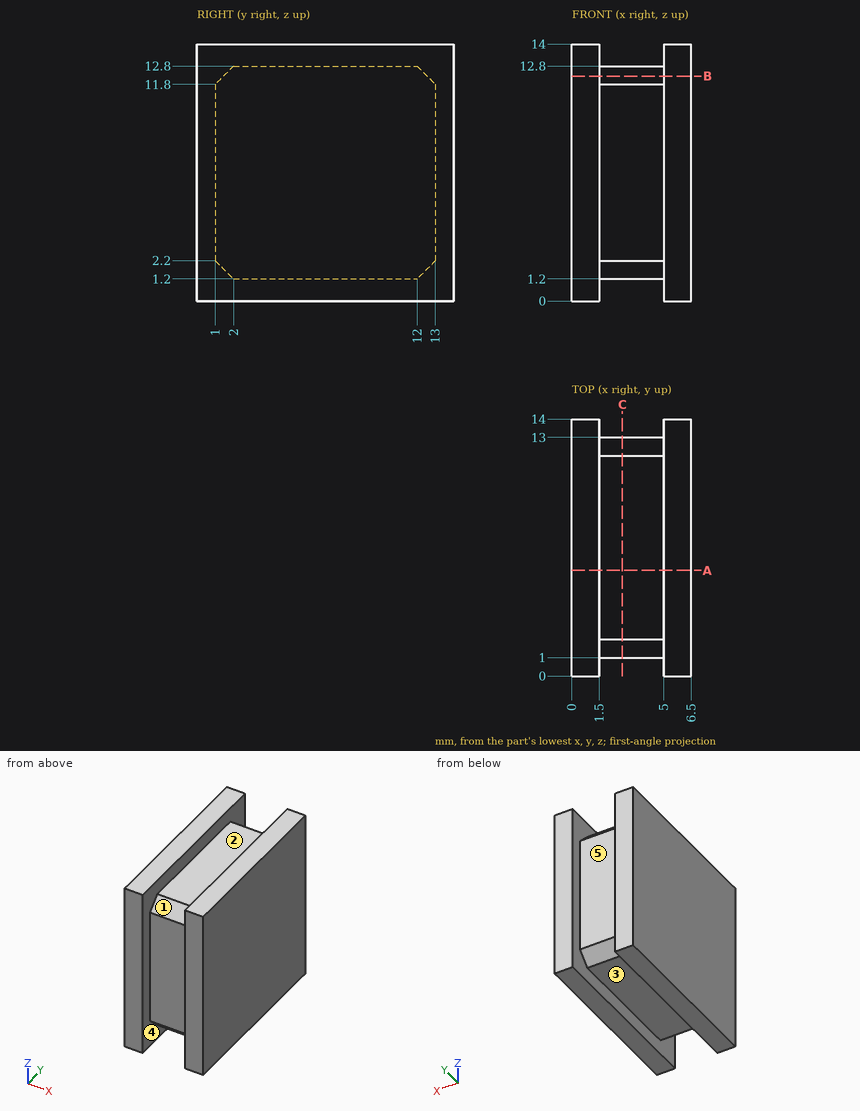
Drawing for the job (mm, zero at the part's lowest x, y, z). A direction names the side the tool comes from. Round coordinates to 2 decimals unless told otherwise and drop trailing zeros. Order: outer loops, then holes, each group sorted by start corner. A loop starts at its lowest first (then second) coordinate and runs counter-clockwise, first axis right, second up. Notation, with made-up numbers: M 58.25,-21 L 68.25,-21 A20 cw 68.25,5 Z; hole C 18.5,27.5 d9. An arc over 180 degrees is marked long. Use one line per item in the form item = value.
Q1. Flat gauge pin, fed straight in: P1, Ø1.8, axis at x = 2.5, y = 5.5, coming from the -Z side. Where does the tip first touch, or does it go through?
Recorded:
P1 = 1.2
Q2. Saw through at C-C on x = 2.75. Give the cut face in (y, z), then the cut area to 3 significant figures.
Recorded:
outline = M 1,2.2 L 2,1.2 L 12,1.2 L 13,2.2 L 13,11.8 L 12,12.8 L 2,12.8 L 1,11.8 Z
area = 137 mm^2
Q3. Saw through at B-B on z = 12.25. Give the cut face in (x, y).
Recorded:
outline = M 0,0 L 1.5,0 L 1.5,1.45 L 5,1.45 L 5,0 L 6.5,0 L 6.5,14 L 5,14 L 5,12.55 L 1.5,12.55 L 1.5,14 L 0,14 Z
Q4. Which spindle directions (+Z, -Z, +X, -X, +Y, -Y) get a long thin tool onto all of the face, cutting with end or side? Do the marked faces 1, 2, 3, 4 and 5. Say none if no direction does.
Recorded:
face_1 = +Z, -Y
face_2 = +Z, +Y, -Y
face_3 = -Z, +Y, -Y
face_4 = none
face_5 = +Z, -Z, +Y
Q5. Probe L1, parallel to Z at x = 4.5, y = 8.75; L2, parallel to Y at x = 2.5, z = 3; L3, parallel to Y at x = 2, z = 1.5. List the from-to ranges inside material, lowest first.
Recorded:
L1 = 1.2 to 12.8
L2 = 1 to 13
L3 = 1.7 to 12.3
Q6. Saw through at A-A on y = 5.75. Give the cut face in (x, z), then the cut area to 3 significant figures.
Recorded:
outline = M 0,0 L 1.5,0 L 1.5,1.2 L 5,1.2 L 5,0 L 6.5,0 L 6.5,14 L 5,14 L 5,12.8 L 1.5,12.8 L 1.5,14 L 0,14 Z
area = 82.6 mm^2
